Read the model definition and answer for the solid it produces. Units are mm, in the model's axes. A direction names the side the tool comes from. Coordinates: 2 decimals unless noted, no trailing zeros. Loops run counter-clockwise (first coordinate to the right, second up) from the corner with the lowest first, then second, coordinate; pieces in that order, holes last.
from build123d import *

# Parameters (mm, degrees)
CHAMFER1_SIZE = 0.5


with BuildPart() as part:
    # Sketch1 → Revolve1 (revolve)
    with BuildSketch(Plane.XY):
        Polygon((1, -10.3), (3, -10.3), (3, -5.3), (1.4, -5.3), (1.4, -3.2), (3.5, -3.2), (3.5, 10.3), (2, 10.3), (2, 6.3), (1, 5.722649731), align=None)
    revolve(axis=Axis((0, -10.3, 0), (0, 1, 0)))

    # Chamfer1
    chamfer1_edges = [part.edges().sort_by_distance(p)[0] for p in [
        (-3.5, 10.3, 0),
    ]]
    chamfer(chamfer1_edges, length=CHAMFER1_SIZE)


solid = part.part
Item 1: A cutting plane is placed at D-D on y = -6.75. Determine the outline of the cut face in (x, z).
Numbers:
outline: circle Ø6 at (0, 0); hole circle Ø2 at (0, 0)
Item 2: Given pin 1 (4 mm diameter, centred on x = -1.5, y = -5, fed in from +Z); pin 2 (2 mm diameter, centred on x = -2.5, y = 2, fed in from -Z); pin 3 (2 mm diameter, centred on y = -5, z = -0.5, fed in from -X), each flat-ended and moving along its own axis, determine where each tip first touches the part or whether it passes through.
Numbers:
pin 1: stops at z = 3.44
pin 2: stops at z = -3.16
pin 3: stops at x = -3
Item 3: A cutting plane is placed at C-C on y = -3.75. Determine the outline of the cut face in (x, z), then the cut area to 3 significant figures.
Numbers:
outline: circle Ø2.8 at (0, 0); hole circle Ø2 at (0, 0)
area: 3.02 mm2
Item 4: A cutting plane is placed at B-B on z = 0. Determine the outline of the cut face in (x, y), then the cut area to 3 significant figures.
Numbers:
outline: (-3.5, -3.2) - (-1.4, -3.2) - (-1.4, -5.3) - (-3, -5.3) - (-3, -10.3) - (-1, -10.3) - (-1, 5.72) - (-2, 6.3) - (-2, 10.3) - (-3, 10.3) - (-3.5, 9.8) - close; (1, -10.3) - (3, -10.3) - (3, -5.3) - (1.4, -5.3) - (1.4, -3.2) - (3.5, -3.2) - (3.5, 9.8) - (3, 10.3) - (2, 10.3) - (2, 6.3) - (1, 5.72) - close
area: 80.4 mm2
Item 5: Find the intervals of material crossed by line 1 along Y through (x, z) = (-2, -2); line 2 along X through (y, z) = (7.45, 0); line 3 along Z through (x, y) = (0, 4.5), in increasing order.
Numbers:
line 1: y = -10.3 to -5.3, -3.2 to 10.3
line 2: x = -3.5 to -2, 2 to 3.5
line 3: z = -3.5 to -1, 1 to 3.5
Item 6: Which of the six approach directions +Z, -Z, +X, -X, +Y, -Y give full straight-line access (tool end or side, diameter ignored) to faces 4 (the face through (1, -10.3, -1)), 5 (the face through (-3, -8, 0)), 6 (the face through (0, 8, 2))?
Numbers:
face 4: +Z, -Z, +X, -X, -Y
face 5: -Y
face 6: +Y
Item 7: A cutting plane is placed at A-A on x = 0. Determine the outline of the cut face in (y, z).
Numbers:
outline: (-10.3, -3) - (-5.3, -3) - (-5.3, -1.4) - (-3.2, -1.4) - (-3.2, -3.5) - (9.8, -3.5) - (10.3, -3) - (10.3, -2) - (6.3, -2) - (5.72, -1) - (-10.3, -1) - close; (-10.3, 1) - (5.72, 1) - (6.3, 2) - (10.3, 2) - (10.3, 3) - (9.8, 3.5) - (-3.2, 3.5) - (-3.2, 1.4) - (-5.3, 1.4) - (-5.3, 3) - (-10.3, 3) - close
Item 8: Determine the mould class of faces 1 (the face through (0, -2, 1)), 2 (the face through (0, -3.2, 2)), 3 (the face through (-1.4, -4.24, -0.06)) for opening direction Z: released by +Z, released by -Z, zero draft, split by the parting line, or undercut.
Numbers:
face 1: undercut
face 2: zero draft
face 3: split by the parting line
